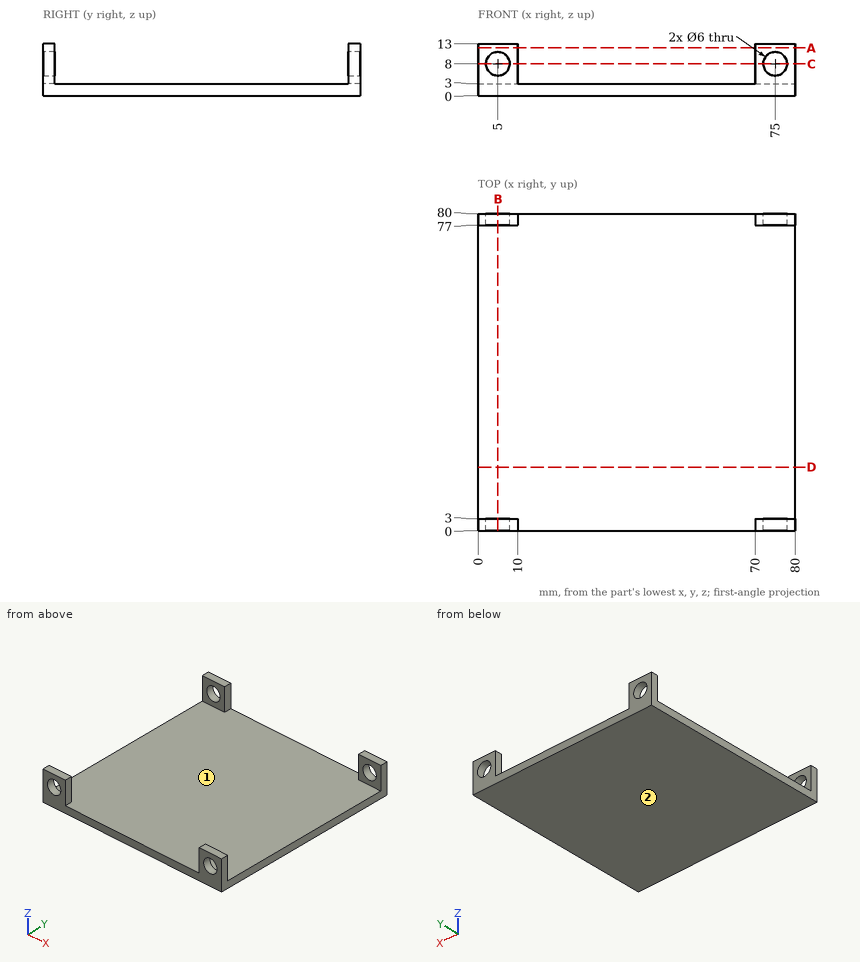
Can you work these out from the drawing? Everything is in mm from the part's minimum corner. Give positions to 0.01 mm unless a question says otherwise; leave off trailing zeros. Order: outer loops, then holes, each group sorted by start corner. A loop starts at its lowest first (then second) coordinate and runs counter-clockwise, first axis right, second up.
Item 1: If we section it at B-B, the plane x = 5: Write out the boundary of the cut face in (y, z).
Item 2: If we section it at A-A, the plane z = 12: Write out the boundary of the cut face in (x, y).
Item 3: If we section it at C-C, the plane z = 8: Count the separate pieces of the cut face and the enclosed holes in it, plus the area to 3 significant figures.
Item 4: If we section it at D-D, the plane y = 16: Write out the boundary of the cut face in (x, z), plus the area to 3 significant figures.
Item 5: I'm going to push a flat-ended pin straight in: pin 1 (1 mm diameter, centred on x = 52.5, y = 22, fed in from +Z). Where does the tip first touch, or does it pass through?
Item 6: If we mould it in two halves opening along Y, with no side actions, what happens to the marked faces 1 and 2? For each: pulls with the +Y half, pulls with the -Y half, needs draft (parallel to the pull), parting line crosses it, or undercut.
Item 7: I need wall thicknesses on line 1 (X direction, y = 2.25, z = 8); line 2 (Y direction, x = 6.5, z = 12.25); line 3 (Z direction, x = 75, y = 1.95). Which ranges of each line are inside material? Lowest first, please.
Values:
1. outline: (0, 0) - (80, 0) - (80, 5) - (77, 5) - (77, 3) - (3, 3) - (3, 5) - (0, 5) - close; (0, 11) - (3, 11) - (3, 13) - (0, 13) - close; (77, 11) - (80, 11) - (80, 13) - (77, 13) - close
2. outline: (0, 0) - (10, 0) - (10, 3) - (0, 3) - close; (0, 77) - (10, 77) - (10, 80) - (0, 80) - close; (70, 0) - (80, 0) - (80, 3) - (70, 3) - close; (70, 77) - (80, 77) - (80, 80) - (70, 80) - close
3. separate pieces: 8
3. enclosed holes: 0
3. area: 48.0 mm2
4. outline: (0, 0) - (80, 0) - (80, 3) - (0, 3) - close
4. area: 240 mm2
5. pin 1: stops at z = 3
6. face 1: undercut
6. face 2: needs draft
7. line 1: x = 0 to 2, 8 to 10, 70 to 72, 78 to 80
7. line 2: y = 0 to 3, 77 to 80
7. line 3: z = 0 to 5, 11 to 13
